Read the model definition and answer for the solid it produces. Units are mm, in the model's axes. A direction names the side the tool comes from. Coordinates: 2 decimals unless noted, no trailing zeros. Loops run counter-clockwise (first coordinate to the right, second up) from the corner with the lowest first, then second, coordinate; pieces in that order, holes last.
Q1. Section A-A (z = 6.5) is taken. Count the separate pieces of the cut face and the enclosed holes in it, then the cut area to 3 significant figures.
Q2. The mould has two halves that part along Y. Classify faces 1 (the face through (-25.48, 27.48, 7.12)), 2 (the face through (-44, 18, 6)), 3 (the face through (-14, 16, 6)), 4 (the face through (-17, 7, 6)): pulls with the +Y half, pulls with the -Y half, needs draft (parallel to the pull), parting line crosses it, or undercut.
Q3. Flat-ended cylindrical pins translate along their axes: P1, Ø4, axis at y = 4, z = 8, coming from the +X side; P2, Ø1.5, axis at x = -16.5, z = 5, coming from the -Y side; P3, Ø0.9, axis at x = -16, y = 4, coming from the +Z side; P4, Ø1.2, axis at x = -42.7, z = 5.9, coming from the +Y side. Find the tip coordinate at first contact, or state that the pin passes through.
Q4. Straight lines are drawn through the part: line 1 (X direction, y = 16.8, z = 5.9); line 2 (Y direction, x = -17, z = 9); line 3 (Y direction, x = -34.5, z = 7). For each, find the intervals that lie inside material, in ascending order.
Q5. Section D-D (x = -38) is taken. Give the vertices of the cut face in (y, z), then the cut area to 3 significant figures.
Q6. Section C-C (z = 4.5) is taken. Give the vertices of the cut face in (x, y).
Q7. Which of the six approach directions +Z, -Z, +X, -X, +Y, -Y give full straight-line access (tool end or side, diameter ignored) to faces 5 (the face through (-17.996, 20, 6)), 6 (the face through (-17, 3, 6)), 7 (the face through (-29.79, 23.97, 5.64))?
Q8. Section B-B (y = 5.25) is taken. Give the vertices of the cut face in (x, z), then the cut area to 3 significant figures.
from build123d import *

# Parameters (mm, degrees)
BOSS_EXTRU_1_DEPTH      = 11.8
ESQUISSE2_R             = 1
ENL_V_MAT_EXTRU_1_DEPTH = 11.8
ESQUISSE3_R             = 5.9
BOSS_EXTRU_2_DEPTH      = 4
ESQUISSE4_R             = 2
BOSS_EXTRU_3_DEPTH      = 3
ESQUISSE5_W             = 5
ESQUISSE5_H             = 4
BOSS_EXTRU_4_DEPTH      = 3


with BuildPart() as part:
    # Esquisse1 → Boss.-Extru.1 (new body)
    with BuildSketch(Plane.XY):
        Polygon((-45.196459949, 18), (-40.196459949, 18), (-40.196459949, 22), (-17.996459949, 22), (-17.996459949, 18), (-12.996459949, 18), (-12.996459949, 16), (-17.996459949, 16), (-17.996459949, 0), (-40.196459949, 0), (-40.196459949, 16), (-45.196459949, 16), align=None)
    extrude(amount=BOSS_EXTRU_1_DEPTH)

    # Esquisse2 → Enlèv. mat.-Extru.1 (cut)
    with BuildSketch(Plane(origin=(0, 18, 0), x_dir=(1, 0, 0), z_dir=(0, 1, 0))):
        with Locations((-42.696459949, -5.9)):
            Circle(ESQUISSE2_R)
        with Locations((-15.496459949, -5.9)):
            Circle(ESQUISSE2_R)
    extrude(amount=-ENL_V_MAT_EXTRU_1_DEPTH, mode=Mode.SUBTRACT)

    # Esquisse3 → Boss.-Extru.2 (add)
    with BuildSketch(Plane(origin=(0, 22, 0), x_dir=(1, 0, 0), z_dir=(0, 1, 0))):
        with Locations((-23.896459949, -5.9)):
            Circle(ESQUISSE3_R)
    extrude(amount=BOSS_EXTRU_2_DEPTH)

    # Esquisse4 → Boss.-Extru.3 (add)
    with BuildSketch(Plane(origin=(0, 26, 0), x_dir=(1, 0, 0), z_dir=(0, 1, 0))):
        with Locations((-23.896459949, -5.9)):
            Circle(ESQUISSE4_R)
    extrude(amount=BOSS_EXTRU_3_DEPTH)

    # Esquisse5 → Boss.-Extru.4 (add)
    with BuildSketch(Plane(origin=(-17.996459949, 0, 0), x_dir=(0, 0, -1), z_dir=(1, 0, 0))):
        with Locations((-5.8, 5)):
            Rectangle(ESQUISSE5_W, ESQUISSE5_H)
    extrude(amount=BOSS_EXTRU_4_DEPTH)


solid = part.part
Numbers:
1. separate pieces: 3
1. enclosed holes: 0
1. area: 572 mm2
2. face 1: needs draft
2. face 2: pulls with the +Y half
2. face 3: undercut
2. face 4: undercut
3. P1: stops at x = -15
3. P2: stops at y = 3
3. P3: stops at z = 8.3
3. P4: passes through
4. line 1: x = -45.2 to -43.7, -41.7 to -16.5, -14.5 to -13
4. line 2: y = 16 to 18
4. line 3: y = 0 to 22
5. outline: (0, 0) - (22, 0) - (22, 11.8) - (0, 11.8) - close
5. area: 260 mm2
6. outline: (-45.2, 16) - (-40.2, 16) - (-40.2, 0) - (-18, 0) - (-18, 3) - (-15, 3) - (-15, 7) - (-18, 7) - (-18, 16) - (-13, 16) - (-13, 18) - (-18, 18) - (-18, 22) - (-18.16, 22) - (-18.16, 26) - (-22.47, 26) - (-22.47, 29) - (-25.32, 29) - (-25.32, 26) - (-29.63, 26) - (-29.63, 22) - (-40.2, 22) - (-40.2, 18) - (-45.2, 18) - close
7. face 5: +Z, -Z, +X, +Y
7. face 6: +Z, -Z, +X, -Y
7. face 7: +Y
8. outline: (-40.2, 0) - (-18, 0) - (-18, 3.3) - (-15, 3.3) - (-15, 8.3) - (-18, 8.3) - (-18, 11.8) - (-40.2, 11.8) - close
8. area: 277 mm2
